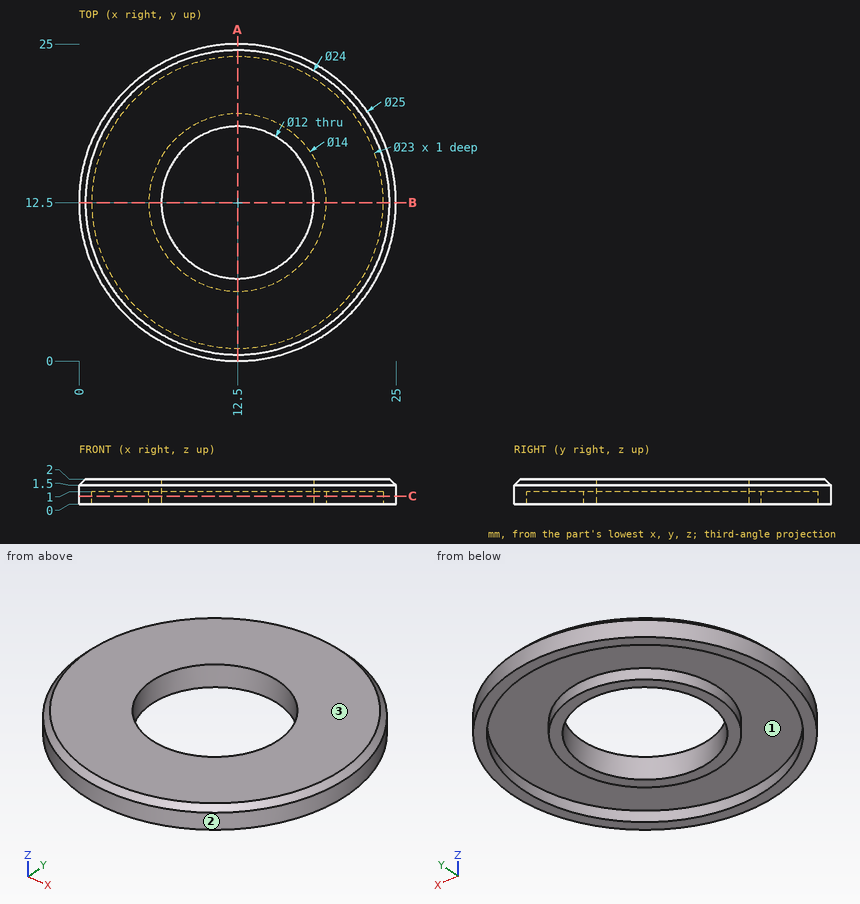
Input: dimensioned drawing with shaded views. Units: mm. Origin: part minimum x, y, z. Give positions to 0.01 mm unless a question says otherwise; leave off trailing zeros. Write each loop counter-clockwise with the first axis right and the second up, starting at its lowest first coordinate (ties: lowest second). Pieces come first, ordered by that corner, then holes.
Q1. Section C-C, the plane z = 0.65. Output: boundary loops of the cut face in (x, y), plus the area to 3 significant figures.
Q2. Pull-direction query (X, two-part tool) for the marked faces 1, 2 and 3; classes: pulls with the +X half, pulls with the -X half, needs draft (parallel to the pull), parting line crosses it, or undercut.
Q3. Section A-A, the plane x = 12.5. Output: boundary loops of the cut face in (y, z), plus the area to 4 significant figures.
Q4. Material intervals for probe 1 along Y at (x, z) = (12.5, 0.5); probe 2 along Y at (x, z) = (12.25, 1.3); probe 3 along X at (y, z) = (16.5, 0.75), sorted ascending.
Filled in:
1. outline: circle Ø25 at (12.5, 12.5); circle Ø14 at (12.5, 12.5); hole circle Ø23 at (12.5, 12.5); hole circle Ø12 at (12.5, 12.5)
1. area: 116 mm2
2. face 1: undercut
2. face 2: parting line crosses it
2. face 3: needs draft
3. outline: (0, 0) - (1, 0) - (1, 1) - (5.5, 1) - (5.5, 0) - (6.5, 0) - (6.5, 2) - (0.5, 2) - (0, 1.5) - close; (18.5, 0) - (19.5, 0) - (19.5, 1) - (24, 1) - (24, 0) - (25, 0) - (25, 1.5) - (24.5, 2) - (18.5, 2) - close
3. area: 16.75 mm2
4. probe 1: y = 0 to 1, 5.5 to 6.5, 18.5 to 19.5, 24 to 25
4. probe 2: y = 0 to 6.51, 18.49 to 25
4. probe 3: x = 0.66 to 1.72, 6.76 to 8.03, 16.97 to 18.24, 23.28 to 24.34
